```python
from build123d import *

# Parameters (mm, degrees)
SKETCH6_R           = 11
BOSS_EXTRUDE3_DEPTH = 2
CHAMFER3_SIZE       = 0.25
SKETCH7_R           = 2
BOSS_EXTRUDE4_DEPTH = 1.5
SKETCH8_R           = 2
CUT_EXTRUDE1_DEPTH  = 26.734218465


with BuildPart() as part:
    # Sketch6 → Boss-Extrude3 (new body)
    with BuildSketch(Plane(origin=(0, 0, 0), x_dir=(1, 0, 0), z_dir=(0, 1, 0))):
        with Locations(Location((0, 0, 0), (0, 0, 270))):
            Circle(SKETCH6_R)
    extrude(amount=BOSS_EXTRUDE3_DEPTH)

    # Chamfer3
    chamfer3_edges = [part.edges().sort_by_distance(p)[0] for p in [
        (0, 0, -11),
        (0, 2, -11),
    ]]
    chamfer(chamfer3_edges, length=CHAMFER3_SIZE)

    # Sketch7 → Boss-Extrude4 (add)
    with BuildSketch(Plane.XY.offset(6)):
        with BuildLine():
            Line((-7, 0), (7, 0))
            Line((7, 0), (-1.91433359, -16.651866461))
            ThreePointArc((-1.91433359, -16.651866461), (-6.021545449, -18.347602858), (-8.482216912, -14.647628922))
            Line((-8.482216912, -14.647628922), (-7, 0))
        make_face()
        with Locations((-5, -15)):
            Circle(SKETCH7_R, mode=Mode.SUBTRACT)
    boss_extrude4 = extrude(amount=BOSS_EXTRUDE4_DEPTH)

    # Mirror2: Boss-Extrude4 across plane
    add(boss_extrude4.mirror(Plane.XY))

    # Sketch8 → Cut-Extrude1 (cut, through all)
    with BuildSketch(Plane(origin=(0, 2, 0), x_dir=(1, 0, 0), z_dir=(0, 1, 0))):
        with Locations(Location((0, 0, 0), (0, 0, 270))):
            Circle(SKETCH8_R)
    extrude(amount=-CUT_EXTRUDE1_DEPTH, mode=Mode.SUBTRACT)


solid = part.part
```
Geometry check sheet. Reference: the model listing, model coordinates, mm. A direction names the side the tool comes from. Give positions to 0.01 mm unless a question says otherwise; leave off trailing zeros. Order: outer loops, then holes, each group sorted by start corner. A loop starts at its lowest first (then second) coordinate and runs counter-clockwise, first axis right, second up.
1. Section check C-C, the plane y = -12. Enter the section's corners in (x, z).
2. Release check for a two-part mould opening along Y. For faces 6 (the face through (0.2, 2, 2.2)), 7 (the face through (-5, -13, 7)), 8 (the face through (2.605, -8.209, -6.74)), 9 (the face through (-2, -7, 6)) record: pulls with the +Y half, pulls with the -Y half, needs draft (parallel to the pull), parting line crosses it, or undercut.
3. Access from +Z, -Z, +X, -X, +Y, -Y to the whole of each face (thin tool, end or side, straight path). Record for faces 1 (the face through (-2, -7, -7.5)), 2 (the face through (-2, -7, -6)), 3 (the face through (-5, -13, -7)), 4 (the face through (-2, -7, 7.5)), 5 (the face through (-7.75, -7.43, 6.74)).
4. Gauge pin test, flat ends, axial feed: pin 1 Ø8 at (x, z) = (3, 7.5) entering from -Y; pin 2 Ø3 at (x, z) = (6.5, -6.5) entering from -Y; pin 3 Ø10 at (x, y) = (4, -13.5) entering from -Z; pin 4 Ø2.5 at (x, z) = (0, 0) entering from +Y. Record the tip position at first contact, or that the pin passes through.
5. Section check B-B, the plane y = -15. Enter the section's corners in (x, z).
6. Section check D-D, the plane x = 0. Enter the section's corners in (y, z), and give its area (3 significant figures).
7. Thickness scan on L1, parallel to Z at x = -2.5, y = -15.75; L2, parallel to Y at x = -5, z = 6.75; L3, parallel to X at y = 1.3, z = 0. Record the ranges inside material, lowest first.
8. Section check A-A, the plane z = 0. Enter the section's corners in (x, y), and give its area (3 significant figures).
Values follow:
1. outline: (-8.21, -7.5) - (0.58, -7.5) - (0.58, -6) - (-8.21, -6) - close; (-8.21, 6) - (0.58, 6) - (0.58, 7.5) - (-8.21, 7.5) - close
2. face 6: pulls with the +Y half
2. face 7: undercut
2. face 8: pulls with the -Y half
2. face 9: needs draft
3. face 1: -Z, +X, -X, -Y
3. face 2: +X, -X, -Y
3. face 3: +Z, -Z
3. face 4: +Z, +X, -X, -Y
3. face 5: +Z, -Z, -X
4. pin 1: stops at y = -14.94
4. pin 2: stops at y = -3.74
4. pin 3: stops at z = -7.5
4. pin 4: passes through
5. outline: (-8.5, -7.5) - (-7, -7.5) - (-7, -6) - (-8.5, -6) - close; (-8.5, 6) - (-7, 6) - (-7, 7.5) - (-8.5, 7.5) - close; (-3, -7.5) - (-1.03, -7.5) - (-1.03, -6) - (-3, -6) - close; (-3, 6) - (-1.03, 6) - (-1.03, 7.5) - (-3, 7.5) - close
6. outline: (-13.08, -7.5) - (0, -7.5) - (0, -10.75) - (0.25, -11) - (1.75, -11) - (2, -10.75) - (2, -2) - (0, -2) - (0, -6) - (-13.08, -6) - close; (-13.08, 6) - (0, 6) - (0, 2) - (2, 2) - (2, 10.75) - (1.75, 11) - (0.25, 11) - (0, 10.75) - (0, 7.5) - (-13.08, 7.5) - close
6. area: 75.1 mm2
7. L1: z = -7.5 to -6, 6 to 7.5
7. L2: y = -18.5 to -17, -13 to 2
7. L3: x = -11 to -2, 2 to 11
8. outline: (-11, 0.25) - (-10.75, 0) - (-2, 0) - (-2, 2) - (-10.75, 2) - (-11, 1.75) - close; (2, 0) - (10.75, 0) - (11, 0.25) - (11, 1.75) - (10.75, 2) - (2, 2) - close
8. area: 35.9 mm2
